For this review, take the finished solid that the model builds, in its own axes (mm). Give positions to 0.01 mm unless a question says otherwise; leave off trailing zeros. Write each loop counter-clockwise with the first axis right and the second up, starting at its lowest first coordinate (ties: lowest second). Pieces come first, ordered by that corner, then holes.
Autodesk Inventor part; units mm, degrees
ref_plane "YZ Plane" through (0, 0, 0) normal (1, 0, 0) x (0, 1, 0)
ref_plane "XZ Plane" through (0, 0, 0) normal (0, 1, 0) x (-1, 0, 0)
ref_plane "XY Plane" through (0, 0, 0) normal (0, 0, 1) x (1, 0, 0)
sketch "Sketch1" plane through (0, 0, 0) normal (0, 1, 0) x (-1, 0, 0)
  circle A0 centre (0, 0) radius 73.025
  line L0 (0, 0) -> (0, -73.025) construction
  line L1 (0, 0) -> (-12.6807, -71.9156)
  line L2 (0, 0) -> (12.6807, -71.9156)
  line L3 (0, 0) -> (72.3143, -10.1631)
  line L4 (0, 0) -> (64.4772, -34.2832)
  line L5 (0, 0) -> (32.0121, 65.6344)
  line L6 (0, 0) -> (52.5298, 50.7274)
  line L7 (0, 0) -> (-52.5298, 50.7274)
  line L8 (0, 0) -> (-32.0121, 65.6344)
  line L9 (0, 0) -> (-64.4772, -34.2832)
  line L10 (0, 0) -> (-72.3143, -10.1631)
  circle A1 centre (0, 0) radius 69.85
  arc A2 (4.7597, -69.6876) -> (-4.7597, -69.6876) centre (0, -69.85) ccw
  arc A3 (67.7477, -17.0079) -> (64.806, -26.0614) centre (66.4313, -21.5848) ccw
  arc A4 (37.1107, 59.1762) -> (44.8121, 53.5808) centre (41.0568, 56.5098) ccw
  arc A5 (-44.8121, 53.5808) -> (-37.1107, 59.1762) centre (-41.0568, 56.5098) ccw
  arc A6 (-64.806, -26.0614) -> (-67.7477, -17.0079) centre (-66.4313, -21.5848) ccw
  point P0 (61.6739, -32.7926)
  point P1 (69.1702, -9.7212)
  point P2 (50.2459, 48.5219)
  point P3 (30.6202, 62.7808)
  point P4 (-30.6202, 62.7808)
  point P5 (-50.2459, 48.5219)
  point P6 (-69.1702, -9.7212)
  point P7 (-61.6739, -32.7926)
  point P8 (-12.1293, -68.7888)
  point P9 (12.1293, -68.7888)
  point P10 (64.806, -26.0614)
  point P11 (67.7477, -17.0079)
  point P12 (44.8121, 53.5808)
  point P13 (37.1107, 59.1762)
  point P14 (-37.1107, 59.1762)
  point P15 (-67.7477, -17.0079)
  dimension "d0" = 146.05
  dimension "d1" = 10
  dimension "d4" = 360
  dimension "d6" = 3.175
  dimension "d10" = 9.525
  dimension "d13" = 360
extrude "Extrusion1" add sketch "Sketch1" along normal blind 1.5875 contours A0 L3 A1 L6 | L5 A1 L8 A0 | A1 L3 L6 | L6 L5 A1 A4 | A0 L2 A1 L4 | A1 A3 L4 L3 | L5 L8 A1 | L2 A1 A2 L1 | L4 A1 L2 | L10 A1 L7 | L7 A1 A5 L8 | L1 A1 L9 | L9 A1 A6 L10 | L7 A1 L10 A0 | L1 A0 L9 A1
fillet "Fillet1" radius 1.5875 30 edges at (30.6202, 0.7937, 62.7808) (32.0121, 0.7937, 65.6344) (-30.6202, 0.7937, 62.7808) (-32.0121, 0.7937, 65.6344) (-52.5298, 0.7937, 50.7274) (-50.2459, 0.7937, 48.5219) (52.5298, 0.7937, 50.7274) (50.2459, 0.7937, 48.5219) (64.4772, 0.7937, -34.2832) (61.6739, 0.7937, -32.7926) (72.3143, 0.7937, -10.1631) (69.1702, 0.7937, -9.7212) (12.6807, 0.7937, -71.9156) (12.1293, 0.7937, -68.7888) (-12.6807, 0.7937, -71.9156) (-12.1293, 0.7937, -68.7888) (-72.3143, 0.7937, -10.1631) (-69.1702, 0.7937, -9.7212) (-64.4772, 0.7937, -34.2832) (-61.6739, 0.7937, -32.7926) (37.1107, 0.7937, 59.1762) (44.8121, 0.7937, 53.5808) (-44.8121, 0.7937, 53.5808) (-37.1107, 0.7937, 59.1762) (-64.806, 0.7937, -26.0614) (-67.7477, 0.7937, -17.0079) (4.7597, 0.7937, -69.6876) (-4.7597, 0.7937, -69.6876) (67.7477, 0.7937, -17.0079) (64.806, 0.7937, -26.0614)
sketch "Sketch5" plane through (0, 1.5875, 0) normal (0, 1, 0) x (1, 0, 0)
  line L0 (0, 0) -> (0, 65.0875) construction
  arc A0 (-4.554, 68.4564) -> (4.554, 68.4564) centre (0, 69.85) ccw
  circle A1 centre (0, 50.8) radius 22.225
  arc A2 (63.6995, 35.7075) -> (14.2757, 71.616) centre (0, 0) ccw
  circle A3 centre (-24.6062, 60.325) radius 1.7526
  circle A4 centre (-24.6062, 60.325) radius 3.175 construction
  circle A5 centre (-22.225, 34.925) radius 3.175
  circle A6 centre (-22.225, 34.925) radius 1.7526
  circle A7 centre (24.6062, 60.325) radius 1.7526
  circle A8 centre (24.6062, 60.325) radius 3.175
  circle A9 centre (22.225, 34.925) radius 3.175
  circle A10 centre (22.225, 34.925) radius 1.7526
  arc A11 (6.2133, 69.5731) -> (4.554, 68.4564) centre (6.0721, 67.9919) ccw
  arc A12 (6.2133, 69.5731) -> (4.554, 68.4564) centre (6.0721, 67.9919) ccw
  arc A13 (-4.554, 68.4564) -> (-6.2133, 69.5731) centre (-6.0721, 67.9919) ccw
  arc A14 (-4.554, 68.4564) -> (-6.2133, 69.5731) centre (-6.0721, 67.9919) ccw
  arc A15 (-12.4019, 70.3348) -> (-10.5977, 69.0414) centre (-10.8385, 70.6105) ccw
  arc A16 (10.5977, 69.0414) -> (12.4019, 70.3348) centre (10.8385, 70.6105) ccw
  arc A17 (10.5977, 69.0414) -> (6.2133, 69.5731) centre (0, 0) ccw
  arc A18 (10.5977, 69.0414) -> (11.9875, 69.515) centre (10.8385, 70.6105) ccw
  arc A19 (-6.2133, 69.5731) -> (-10.5977, 69.0414) centre (0, 0) ccw
  arc A20 (-14.2757, 71.616) -> (-63.6995, 35.7075) centre (0, 0) ccw
  line L1 (-28.4451, 67.2572) -> (-25.3861, 34.6286)
  line L2 (-22.7046, 31.7864) -> (-3.3572, 28.83)
  line L3 (28.4451, 67.2572) -> (25.3861, 34.6286)
  line L4 (22.7046, 31.7864) -> (3.3572, 28.83)
  circle A21 centre (0, 0) radius 73.025
  circle A22 centre (0, 50.8) radius 19.05
  point P0 (-63.6995, 35.7075)
  point P1 (-9.2869, 69.2299)
  point P2 (9.2869, 69.2299)
  point P3 (-5.0165, 69.1776)
  point P4 (5.0165, 69.1776)
  dimension "d40" = 44.45
  dimension "d41" = 3.5052
  dimension "d42" = 6.35
  dimension "d43" = 9.525
  dimension "d44" = 24.6062
  dimension "d45" = 6.35
  dimension "d46" = 3.5052
  dimension "d47" = 15.875
  dimension "d48" = 22.225
  dimension "d70" = 38.1
extrude "Extrusion3" cut sketch "Sketch5" against normal blind 25.4 contours A13 A22 A11 A0 | A0 A11 A22 A13 | A1 L4 A9 L3 A2 A21 A20 L1 A5 L2 | A3 | A6 | A7 | A10
fillet "Fillet4" radius 6.35 2 edges at (-28.4451, 0.7937, -67.2572) (28.4451, 0.7937, -67.2572)
fillet "Fillet5" radius 3.175 2 edges at (-5.0163, 0.7937, -69.1777) (5.0163, 0.7937, -69.1777)
equation "\"d45\" = d42"
equation "\"d46\" = d41"
properties part number "Top Plate" material "Aluminum 6061"
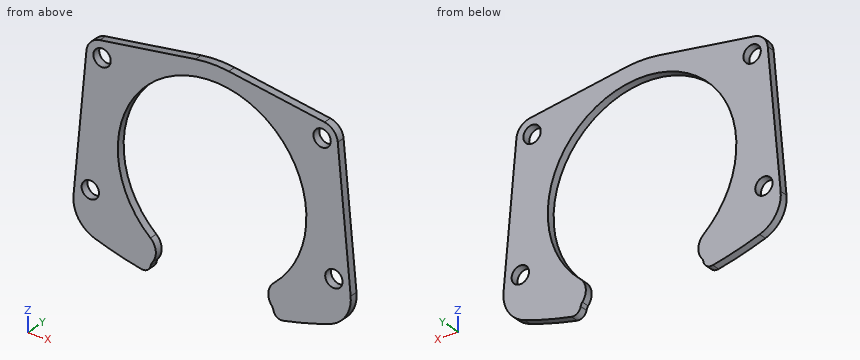
(1) We need section A-A (x = 18). Write out the cut boundary in (y, z), and give its area (3 significant figures).
(2) For L1, parallel to X at y = 1.2, z = -60; L2, parallel to X at y = 0.6, z = -50.8; L3, parallel to X at y = 1, z = -44.5, list the stretches that pass through material, from the lowest coordinate up.
(3) Clearance check with flat-ended pins moving along their axes: pin 1 Ø4.5 at (x, z) = (22.225, -34.925) entering from -Y; pin 2 Ø3 at (x, z) = (-24.61, -60.32) entering from +Y. State where each tip first meets the part, or that it passes through.
(4) We need section C-C (y = 1). Count the separate pieces of the cut face and the enclosed holes in it, and give its area (3 significant figures).
(5) We need section B-B (z = -50.8). Write out the cut boundary in (x, y).
The answers:
1. outline: (0, -70.77) - (1.59, -70.77) - (1.59, -57.04) - (0, -57.04) - close; (0, -44.56) - (1.59, -44.56) - (1.59, -31.07) - (0, -31.07) - close
1. area: 43.2 mm2
2. L1: x = -27.76 to -26.33, -22.88 to -16.68, 16.68 to 22.88, 26.33 to 27.76
2. L2: x = -26.9 to -19.05, 19.05 to 26.9
2. L3: x = -26.31 to -17.98, 17.98 to 26.31
3. pin 1: stops at y = 0
3. pin 2: passes through
4. separate pieces: 1
4. enclosed holes: 4
4. area: 907 mm2
5. outline: (-26.9, 0) - (-19.05, 0) - (-19.05, 1.59) - (-26.9, 1.59) - close; (19.05, 0) - (26.9, 0) - (26.9, 1.59) - (19.05, 1.59) - close
